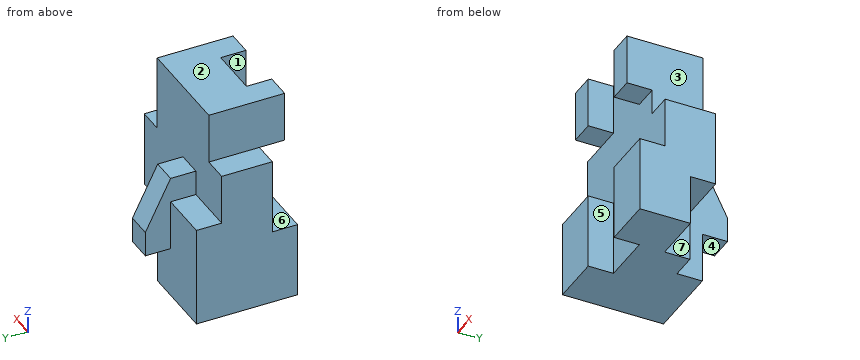
```python
from build123d import *

# Parameters (mm, degrees)
SKETCH1_W           = 6
SKETCH1_H           = 4
BOSS_EXTRUDE1_DEPTH = 8
SKETCH2_W           = 2
SKETCH2_H           = 1
CUT_EXTRUDE1_DEPTH  = 9
SKETCH3_W           = 1
SKETCH3_H           = 2
SKETCH3_H_2         = 3
CUT_EXTRUDE2_DEPTH  = 5
SKETCH4_W           = 3
SKETCH4_H           = 1
CUT_EXTRUDE3_DEPTH  = 7
SKETCH5_OUTSIDE_W   = 10.154
SKETCH5_OUTSIDE_H   = 12.154
CUT_EXTRUDE4_DEPTH  = 1
SKETCH6_W           = 2
SKETCH6_H           = 2
CUT_EXTRUDE5_DEPTH  = 1
SKETCH7_W           = 1
SKETCH7_H           = 3
BOSS_EXTRUDE2_DEPTH = 1
CUT_EXTRUDE6_DEPTH  = 4


with BuildPart() as part:
    # Sketch1 → Boss-Extrude1 (new body)
    with BuildSketch(Plane.XY):
        Rectangle(SKETCH1_W, SKETCH1_H)
    extrude(amount=BOSS_EXTRUDE1_DEPTH)

    # Sketch2 → Cut-Extrude1 (cut, through all)
    with BuildSketch(Plane.XY.offset(8)):
        with Locations((0, -1.5)):
            Rectangle(SKETCH2_W, SKETCH2_H)
    extrude(amount=-CUT_EXTRUDE1_DEPTH, mode=Mode.SUBTRACT)

    # Sketch3 → Cut-Extrude2 (cut, through all)
    with BuildSketch(Plane(origin=(0, 2, 0), x_dir=(1, 0, 0), z_dir=(0, 1, 0))):
        with Locations((-2.5, -7)):
            Rectangle(SKETCH3_W, SKETCH3_H)
        with Locations((2.5, -6.5)):
            Rectangle(SKETCH3_W, SKETCH3_H_2)
    extrude(amount=-CUT_EXTRUDE2_DEPTH, mode=Mode.SUBTRACT)

    # Sketch4 → Cut-Extrude3 (cut, through all)
    with BuildSketch(Plane(origin=(3, 0, 0), x_dir=(0, 0, -1), z_dir=(1, 0, 0))):
        with Locations((-4.5, -1.5)):
            Rectangle(SKETCH4_W, SKETCH4_H)
    extrude(amount=-CUT_EXTRUDE3_DEPTH, mode=Mode.SUBTRACT)

    # Sketch5 outside → Cut-Extrude4 (cut)
    with BuildSketch(Plane(origin=(0, 2, 0), x_dir=(1, 0, 0), z_dir=(0, 1, 0))):
        with Locations((0, -4)):
            Rectangle(SKETCH5_OUTSIDE_W, SKETCH5_OUTSIDE_H)
        Polygon((-3, 0), (0, 0), (0, -5), (-1, -5), (-1, -4), (-3, -4), align=None, mode=Mode.SUBTRACT)
    extrude(amount=-CUT_EXTRUDE4_DEPTH, mode=Mode.SUBTRACT)

    # Sketch6 → Cut-Extrude5 (cut)
    with BuildSketch(Plane(origin=(0, 1, 0), x_dir=(1, 0, 0), z_dir=(0, 1, 0))):
        with Locations((2, -1)):
            Rectangle(SKETCH6_W, SKETCH6_H)
    extrude(amount=-CUT_EXTRUDE5_DEPTH, mode=Mode.SUBTRACT)

    # Sketch7 → Boss-Extrude2 (add)
    with BuildSketch(Plane(origin=(0, 2, 0), x_dir=(1, 0, 0), z_dir=(0, 1, 0))):
        with Locations((-0.5, -3.5)):
            Rectangle(SKETCH7_W, SKETCH7_H)
    extrude(amount=BOSS_EXTRUDE2_DEPTH)

    # Sketch8 → Cut-Extrude6 (cut, through all)
    with BuildSketch(Plane(origin=(0, 0, 0), x_dir=(0, 0, -1), z_dir=(1, 0, 0))):
        Polygon((-3, 3), (-5, 2), (-5, 3), align=None)
    extrude(amount=-CUT_EXTRUDE6_DEPTH, mode=Mode.SUBTRACT)


solid = part.part
```
The listing builds one solid part. Answer for the finished solid, in the listing's coordinates (mm). Face numbers are marked on the shaded views. A direction names the side the tool comes from. Round coordinates to 2 decimals unless told otherwise and drop trailing zeros. Loops run counter-clockwise (first coordinate to the right, second up) from the corner with the lowest first, then second, coordinate; pieces in that order, holes last. Notation, with made-up numbers: (88, -37.75) - (108, -37.75) arc R31 cw to (108, -5.75) - close; hole circle Ø1 at (-30, 8.5). An arc over 180 degrees is marked (long way). Return JSON: item names as keys, results as strings. Group by question number.
1. The part is cut by section B-B on z = 2.25. Determine the outline of the cut face in (x, y).
2. Consider probe 1 along Z at (x, y) = (-1.9, -1.3); probe 2 along Y at (x, z) = (1.6, 7.25); probe 3 along X at (y, z) = (-1.35, 2.25). Determine where each line is inside the solid, lowest interval first.
3. Which of the six approach directions +Z, -Z, +X, -X, +Y, -Y give full straight-line access (tool end or side, diameter ignored) to the marked faces 4, 5, 6 and 7?
4. Each of these flat-tipped pins is pushed along its axis until it touches: P1, Ø1.6, axis at y = 0, z = 7, coming from the -X side; P2, Ø0.8, axis at x = -2.5, y = 1.5, coming from the +Z side; P3, Ø0.8, axis at y = 0.5, z = 1.5, coming from the +X side. Where does it stop, or does it pass through?
5. The part is cut by section C-C on y = -0.9. Determine the outline of the cut face in (x, z).
6. The mould has two halves that part along X. Classify the marked faces 1, 2 and 3: pulls with the +X half, pulls with the -X half, needs draft (parallel to the pull), parting line crosses it, or undercut.
7. The part is cut by section A-A on x = -1.7. Determine the outline of the cut face in (y, z).
8. The part is cut by section D-D on x = -2.45. Determine the outline of the cut face in (y, z), then the cut area to 3 significant figures.
Resolved:
{
 "1": {"outline": "(-3, -2) - (-1, -2) - (-1, -1) - (1, -1) - (1, -2) - (3, -2) - (3, 1) - (0, 1) - (0, 3) - (-1, 3) - (-1, 2) - (-3, 2) - close"},
 "2": {"probe 1": "z = 0 to 3, 6 to 8", "probe 2": "y = -2 to 1", "probe 3": "x = -3 to -1, 1 to 3"},
 "3": {"face 4": "-Z, +X, -X, +Y", "face 5": "+Z, -Z, -Y", "face 6": "+X, -X, -Y", "face 7": "-Z, +X, +Y"},
 "4": {"P1": "stops at x = -2", "P2": "stops at z = 4", "P3": "stops at x = 1"},
 "5": {"outline": "(-3, 0) - (3, 0) - (3, 5) - (2, 5) - (2, 8) - (-2, 8) - (-2, 6) - (-3, 6) - close"},
 "6": {"face 1": "undercut", "face 2": "needs draft", "face 3": "pulls with the +X half"},
 "7": {"outline": "(-2, 0) - (2, 0) - (2, 4) - (1, 4) - (1, 8) - (-2, 8) - (-2, 6) - (-1, 6) - (-1, 3) - (-2, 3) - close"},
 "8": {"outline": "(-2, 0) - (2, 0) - (2, 4) - (1, 4) - (1, 6) - (-1, 6) - (-1, 3) - (-2, 3) - close", "area": "19.0 mm²"}
}
